```python
from build123d import *

# Parameters (mm, degrees)
AUFSATZ_LINEAR_AUSTRAGEN2_DEPTH = 6


with BuildPart() as part:
    # Skizze1 → Aufsatz-Linear austragen2 (new body)
    with BuildSketch(Plane.XY):
        Polygon((30, 0), (0, 30), (-6, 30), (-6, 40), (0, 40), (0, 50), (-6, 50), (-6, 60), (0, 60), (0, 70), (-6, 70), (-6, 80), (0, 80), (0, 90), (-6, 90), (-6, 100), (0, 100), (0, 110), (-6, 110), (-6, 120), (0, 120), (0, 130), (-6, 130), (-6, 140), (0, 140), (0, 150), (-6, 150), (-6, 160), (0, 160), (0, 170), (-6, 170), (-6, 180), (0, 180), (0, 190), (-6, 190), (-6, 200), (0, 200), (0, 210), (-6, 210), (-6, 220), (0, 220), (30, 250), (40, 250), (40, 256), (50, 256), (50, 250), (60, 250), (60, 256), (70, 256), (70, 250), (80, 250), (80, 256), (90, 256), (90, 250), (100, 250), (100, 256), (110, 256), (110, 250), (120, 250), (120, 256), (130, 256), (130, 250), (140, 250), (140, 256), (150, 256), (150, 250), (160, 250), (160, 256), (170, 256), (170, 250), (180, 250), (180, 256), (190, 256), (190, 250), (200, 250), (200, 256), (210, 256), (210, 250), (220, 250), (220, 256), (230, 256), (230, 250), (240, 250), (240, 256), (250, 256), (250, 250), (260, 250), (260, 256), (270, 256), (270, 250), (300, 220), (306, 220), (306, 210), (300, 210), (300, 200), (306, 200), (306, 190), (300, 190), (300, 180), (306, 180), (306, 170), (300, 170), (300, 160), (306, 160), (306, 150), (300, 150), (300, 140), (306, 140), (306, 130), (300, 130), (300, 120), (306, 120), (306, 110), (300, 110), (300, 100), (306, 100), (306, 90), (300, 90), (300, 80), (306, 80), (306, 70), (300, 70), (300, 60), (306, 60), (306, 50), (300, 50), (300, 40), (306, 40), (306, 30), (300, 30), (270, 0), (270, -6), (260, -6), (260, 0), (250, 0), (250, -6), (240, -6), (240, 0), (230, 0), (230, -6), (220, -6), (220, 0), (210, 0), (210, -6), (200, -6), (200, 0), (190, 0), (190, -6), (180, -6), (180, 0), (170, 0), (170, -6), (160, -6), (160, 0), (150, 0), (150, -6), (140, -6), (140, 0), (130, 0), (130, -6), (120, -6), (120, 0), (110, 0), (110, -6), (100, -6), (100, 0), (90, 0), (90, -6), (80, -6), (80, 0), (70, 0), (70, -6), (60, -6), (60, 0), (50, 0), (50, -6), (40, -6), (40, 0), align=None)
        Polygon((30, 190), (60, 220), (240, 220), (270, 190), (270, 60), (240, 30), (60, 30), (30, 60), align=None, mode=Mode.SUBTRACT)
    extrude(amount=AUFSATZ_LINEAR_AUSTRAGEN2_DEPTH)


solid = part.part
```
Input: part model. Units: mm. Frame: model coordinates. A direction names the side the tool comes from. Coordinates: 2 decimals unless noted, no trailing zeros. Write each loop counter-clockwise with the first axis right and the second up, starting at its lowest first coordinate (ties: lowest second). Pieces come first, ordered by that corner, then holes. Notation, with made-up numbers: (70, 72) - (97, 72) arc R12 cw to (97, 78) - close; hole circle Ø7 at (9, -23.75). An arc over 180 degrees is marked (long way). Put each result on its own line as item: value. Start each with the question number.
1) Reachability of faces 4 (the face through (45, 45, 3)), 5 (the face through (285, 15, 3)) from +Z, -Z, +X, -X, +Y, -Y: full face, straight path, thin tool, end or side. Return the list, or none.
2) Cut plane A-A (y = 186.5). Return the cut outline in (x, z).
3) Contact query for flat-ended pins moving along their axis: pin 1 (1.8 mm diameter, centred on x = -1.5, z = 3.5, fed in from -Y); pin 2 (3 mm diameter, centred on x = 134, z = 2, fed in from -Y); pin 3 (1.8 mm diameter, centred on y = 44.5, z = 3, fed in from +X). Output: stop coordinate, or through.
4) Cut plane B-B (x = 175). Return the cut outline in (y, z), plus the area to 3 significant figures.
5) Ray query, L1, parallel to Y at x = 229, z = 2.9; L2, parallel to Y at x = 94.5, z = 0.7; L3, parallel to X at y = 149, z = 3.25. Return the intervals inside material, ascending.
6) Mould query, pull axis X, two halves, no side actions, for faces 1 (the face through (45, 205, 3)), 2 (the face through (285, 235, 3)), 3 (the face through (15, 15, 3)). Classes: pulls with the +X half, pulls with the -X half, needs draft (parallel to the pull), parting line crosses it, or undercut.
Resolved:
1. face 4: +Z, -Z
1. face 5: +Z, -Z, +X, -Y
2. outline: (0, 0) - (30, 0) - (30, 6) - (0, 6) - close; (270, 0) - (300, 0) - (300, 6) - (270, 6) - close
3. pin 1: stops at y = 30
3. pin 2: stops at y = 0
3. pin 3: stops at x = 300
4. outline: (0, 0) - (30, 0) - (30, 6) - (0, 6) - close; (220, 0) - (250, 0) - (250, 6) - (220, 6) - close
4. area: 360 mm2
5. L1: y = -6 to 30, 220 to 256
5. L2: y = 0 to 30, 220 to 250
5. L3: x = 0 to 30, 270 to 300
6. face 1: undercut
6. face 2: pulls with the +X half
6. face 3: pulls with the -X half
